Design review of the part shown in the three views and the two pictorial views. Dimensions are in mm from the part's minimum x, y and z. A direction names the side the tool comes from. Round coordinates to 2 decimals unless told otherwise and drop trailing zeros. Loops run counter-clockwise (first coordinate to the right, second up) from the corner with the lowest first, then second, coordinate; pieces in that order, holes last. Notation, with made-up numbers: (49.5, 61.5) -> (59.5, 61.5) arc R29 ccw to (59.5, 98.5) -> close; hole circle Ø10 at (-14, 79). An arc over 180 degrees is marked (long way). One line per question, with ' | ' between items. Start each with the question number.
1. Consider section D-D (x = 40.5). Write out the cut boundary in (y, z).
2. Draft analysis for pull direction Y (two halves, no side actions). For the marked faces 1, 2 and 3, state which applies: pulls with the +Y half, pulls with the -Y half, needs draft (parallel to the pull), parting line crosses it, or undercut.
3. Consider section B-B (y = 6). Write out the cut boundary in (x, z).
4. Consider section A-A (x = 14.5). Write out the cut boundary in (y, z).
5. Consider section C-C (x = 4). Write out the cut boundary in (y, z) (1 decimal), and give its area (3 significant figures).
6. Wall thickness on line 1 along Y through (x, z) = (12, 34); line 2 along Y through (x, z) = (12.5, 63.5) (1 decimal); line 3 along Z through (x, y) = (17, 13.5): over which ranges is each line inside the solid? List them lowest first.
7. For the marked faces 4 and 5, list the 3-axis set-ups (+Z, -Z, +X, -X, +Y, -Y) from which the entire face can be reached by the end or side of a thin tool; tool diameter is ignored.
8. For pin 1 Ø12 at (x, z) = (33.5, 42.5) entering from +Y (1 decimal); pin 2 Ø4 at (y, z) = (37, 63) entering from -X; pin 3 Ø3 at (x, z) = (45.5, 48) entering from +Y; pin 4 Ø13 at (x, y) = (12.5, 30) entering from -Z, all flat-tipped, find the tip position at first contact; note any pin that passes through.
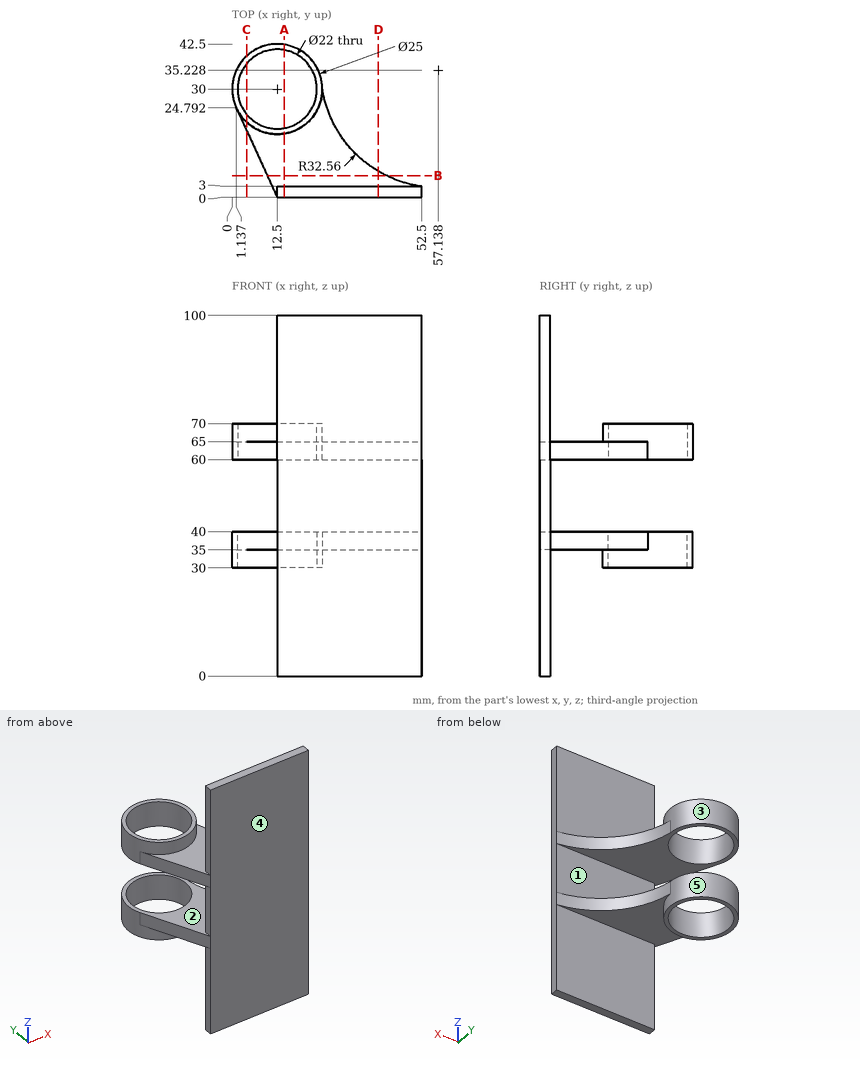
Answer block:
1) outline: (0, 0) -> (3, 0) -> (3, 35) -> (7.24, 35) -> (7.24, 40) -> (3, 40) -> (3, 60) -> (7.24, 60) -> (7.24, 65) -> (3, 65) -> (3, 100) -> (0, 100) -> close
2) face 1: pulls with the +Y half | face 2: needs draft | face 3: undercut
3) outline: (9.75, 35) -> (42.79, 35) -> (42.79, 40) -> (9.75, 40) -> close; (9.75, 60) -> (42.79, 60) -> (42.79, 65) -> (9.75, 65) -> close
4) outline: (0, 0) -> (3, 0) -> (3, 35) -> (17.66, 35) -> (17.66, 30) -> (19.18, 30) -> (19.18, 40) -> (3, 40) -> (3, 60) -> (19.18, 60) -> (19.18, 70) -> (17.66, 70) -> (17.66, 65) -> (3, 65) -> (3, 100) -> (0, 100) -> close; (40.82, 30) -> (42.34, 30) -> (42.34, 40) -> (40.82, 40) -> close; (40.82, 60) -> (42.34, 60) -> (42.34, 70) -> (40.82, 70) -> close
5) outline: (18.5, 35) -> (20.8, 35) -> (20.8, 30) -> (23, 30) -> (23, 40) -> (18.5, 40) -> close; (18.5, 60) -> (23, 60) -> (23, 70) -> (20.8, 70) -> (20.8, 65) -> (18.5, 65) -> close; (37, 30) -> (39.2, 30) -> (39.2, 40) -> (37, 40) -> close; (37, 60) -> (39.2, 60) -> (39.2, 70) -> (37, 70) -> close | area: 110 mm2
6) line 1: y = 17.51 to 19.01, 40.99 to 42.49 | line 2: y = 0 to 19, 41 to 42.5 | line 3: z = 35 to 40, 60 to 65
7) face 4: +Z, -Z, +X, -X, -Y | face 5: -Z
8) pin 1: stops at y = 20.6 | pin 2: stops at x = 1.04 | pin 3: stops at y = 3 | pin 4: passes through
